```python
from build123d import *

# Parameters (mm, degrees)
F0_W     = 10
F0_H     = 50
F2_ANGLE = -75


with BuildPart() as f1:
    # F0 (on Top) → F1 (revolve)
    with BuildSketch(Plane.XY):
        with Locations((-5, 25)):
            Rectangle(F0_W, F0_H)
        with BuildLine():
            Line((0, 50), (0, 0))
            Line((0, 0), (55, 0))
            ThreePointArc((55, 0), (40.355339, 35.355339), (5, 50))
            Line((5, 50), (0, 50))
        make_face()
        Polygon((-10, 50), (0, 50), (-2.608035, 52.608035), (-7.391965, 52.608035), align=None)
    revolve(axis=Axis((27.5, 0, 0), (1, 0, 0)))

    # F0 (on Top) → F2 (revolve)
    with BuildSketch(Plane.XY):
        Polygon((-50.859153, -50), (-10, -50), (-10, -47.028106), (-51.016824, -47.028106), (-86.745456, -42.243611), (-86.745456, -45.194391), align=None)
    revolve(axis=Axis((27.5, 0, 0), (1, 0, 0)), revolution_arc=F2_ANGLE)


solid = f1.part
```
Verification items for the finished model (mm, model axes). A direction names the side the tool comes from. Give positions to 0.01 mm unless a question says otherwise; leave off trailing zeros. Write each loop counter-clockwise with the first axis right and the second up, starting at its lowest first coordinate (ties: lowest second). Pieces come first, ordered by that corner, then holes. Notation, with made-up numbers: (69.5, 49) - (83.5, 49) arc R18 ccw to (83.5, 66) - close; hole circle Ø3 at (52.5, 85). An arc over 180 degrees is marked (long way). Put each result on its own line as item: value.
Q1. Scan lines: probe 1 along X at (y, z) = (5, 29); probe 2 along Z at (x, y) = (35.5, -17); probe 3 along X at (y, z) = (36, -20). Record each from-to range of solid material in increasing order. Write a range as from..to.
Result:
probe 1: -10..45.42
probe 2: -35.79..35.79
probe 3: -10..33.35
Q2. Section check B-B on x = -56. Record the cut outline in (y, z), and give its area (3 significant figures).
Result:
outline: (-49.31, 0) - (-46.36, 0) arc R46.36 cw to (-12, 44.78) - (-12.76, 47.63) arc R49.31 ccw to start
area: 185 mm2
Q3. Depth check by flat-ended pin: P1, Ø3, axis at x = 16.5, z = 9, coming from the +Y side; P2, Ø10, axis at y = -10, z = -27, coming from the +X side; P3, Ø2, axis at x = 9, y = 19, coming from the +Z side. Enter the tip coordinate at first touch or a pass-through.
Result:
P1: y = 48.25
P2: x = 48.98
P3: z = 46.48
Q4. Set-up check for faces 5 (the face through (-48.55, -12.38, 46.2)), 6 (the face through (-9.873, -10.866, -48.935)), 7 (the face through (-30, -40, 30)), 8 (the face through (-49, -48, 0)): record each of +Z, -Z, +X, -X, +Y, -Y from which the full face is reachable in a straight line by a thin tool's end or side.
Result:
face 5: +Z, -X, +Y
face 6: -X
face 7: +Z, -X, -Y
face 8: -Z, -X, +Y, -Y
Q5. Mould release check, pull along X, two halves, no side actions. Record for faces 1 (the face through (-69.13, -35.63, 26.83)), 2 (the face through (2.46, 47.69, 15.02)), 3 (the face through (-68.55, -38.05, 28.65)), 4 (the face through (-30.8, -37.57, 28.29)): released by +X, released by -X, zero draft, split by the parting line, or undercut.
Result:
face 1: undercut
face 2: zero draft
face 3: released by -X
face 4: undercut
Q6. Section check A-A on x = -20.5. Record the cut outline in (y, z), and give its area (3 significant figures).
Result:
outline: (-50, 0) - (-47.03, 0) arc R47.03 cw to (-12.17, 45.43) - (-12.94, 48.3) arc R50 ccw to start
area: 189 mm2
